Source: CAD feature listing. Evaluate the final solid. Frame: model axes, mm. Face numbers are marked on the shaded views. A direction names the side the tool comes from. Coordinates: 2 decimals unless noted, no trailing zeros. Order: outer loops, then holes, each group sorted by start corner. A loop starts at its lowest first (then second) coordinate and runs counter-clockwise, first axis right, second up.
Item 1: Section C-C on z = 28.25. Return the cut outline in (x, y), then the cut area to 3 significant figures.
Item 2: Contact query for flat-ended pins moving along their axis: P1, Ø0.8, axis at x = 15, y = 6.5, coming from the +Z side; P2, Ø1, axis at y = 9, z = 17.5, coming from the +X side; P3, Ø1, axis at x = 15.5, y = 9, coming from the -Z side. Output: stop coordinate, or through.
Item 3: Ray query, line 1 (X direction, y = 8, z = 8); line 2 (Z direction, x = 13.25, y = 6.8); line 3 (Z direction, x = 17.75, y = 8.85). Return the intervals inside material, ascending.
Item 4: Reachability of the marked faces 4, 5, 6 and 7 from +Z, -Z, +X, -X, +Y, -Y: full face, straight path, thin tool, end or side. Return the list, or none.
Item 5: Section B-B on x = 13.25. Return the cut outline in (y, z).
Item 6: Section A-A on y = 8.75. Return the cut outline in (x, z), then the cut area to 3 significant figures.
Item 7: Mould query, pull axis Y, two halves, no side actions, for the marked faces 1, 2 and 3. Classes: released by +Y, released by -Y, zero draft, split by the parting line, or undercut.
Item 8: Section D-D on y = 7.7. Return the cut outline in (x, z).
from build123d import *

# Parameters (mm, degrees)
CYLINDER_R     = 1.5
CYLINDER_DEPTH = 10
BOX004_W       = 1
BOX004_H       = 3
BOX004_DEPTH   = 3
BOX005_W       = 1
BOX005_H       = 3
BOX005_DEPTH   = 3
BOX006_W       = 6
BOX006_H       = 1
BOX006_DEPTH   = 3
BOX007_W       = 6
BOX007_H       = 1
BOX007_DEPTH   = 3
BOX003_W       = 6
BOX003_H       = 3.5
BOX003_DEPTH   = 20


with BuildPart() as cylinder:
    # Cylinder → Cylinder (new body)
    with BuildSketch(Plane(origin=(15, 8.75, 20), x_dir=(1, 0, 0), z_dir=(0, 0, 1))):
        Circle(CYLINDER_R)
    extrude(amount=CYLINDER_DEPTH)


with BuildPart() as box004:
    # Box004 → Box004 (new body)
    with BuildSketch(Plane(origin=(11, 7.25, 7), x_dir=(1, 0, 0), z_dir=(0, 0, 1))):
        with Locations((0.5, 1.5)):
            Rectangle(BOX004_W, BOX004_H)
    extrude(amount=BOX004_DEPTH)


with BuildPart() as box005:
    # Box005 → Box005 (new body)
    with BuildSketch(Plane(origin=(18, 7.25, 7), x_dir=(1, 0, 0), z_dir=(0, 0, 1))):
        with Locations((0.5, 1.5)):
            Rectangle(BOX005_W, BOX005_H)
    extrude(amount=BOX005_DEPTH)


with BuildPart() as box006:
    # Box006 → Box006 (new body)
    with BuildSketch(Plane(origin=(12, 6, 7), x_dir=(1, 0, 0), z_dir=(0, 0, 1))):
        with Locations((3, 0.5)):
            Rectangle(BOX006_W, BOX006_H)
    extrude(amount=BOX006_DEPTH)


with BuildPart() as box007:
    # Box007 → Box007 (new body)
    with BuildSketch(Plane(origin=(12, 10.5, 7), x_dir=(1, 0, 0), z_dir=(0, 0, 1))):
        with Locations((3, 0.5)):
            Rectangle(BOX007_W, BOX007_H)
    extrude(amount=BOX007_DEPTH)


with BuildPart() as bt_ex1:
    # Box003 → Box003 (new body)
    with BuildSketch(Plane(origin=(12, 7, 9), x_dir=(1, 0, 0), z_dir=(0, 0, 1))):
        with Locations((3, 1.75)):
            Rectangle(BOX003_W, BOX003_H)
    extrude(amount=BOX003_DEPTH)

    # Fusion: union Box004, Box005, Box006, Box007
    add(box004.part)
    add(box005.part)
    add(box006.part)
    add(box007.part)

    # Fusion005: union Cylinder
    add(cylinder.part)


solid = bt_ex1.part
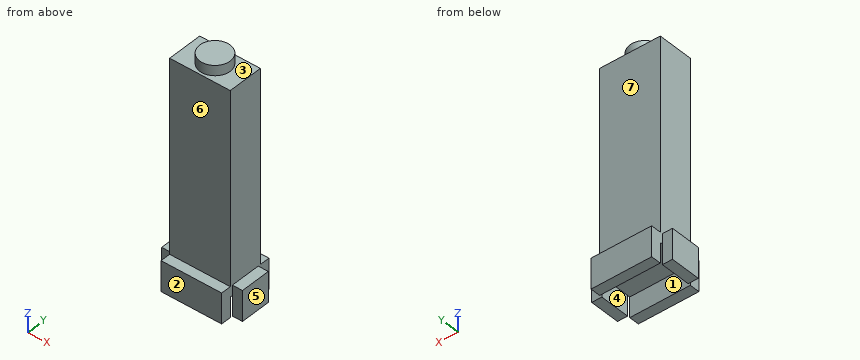
Answer list:
1. outline: (12, 7) - (18, 7) - (18, 10.5) - (12, 10.5) - close
1. area: 21.0 mm2
2. P1: stops at z = 10
2. P2: stops at x = 18
2. P3: stops at z = 9
3. line 1: x = 11 to 12, 18 to 19
3. line 2: z = 7 to 10
3. line 3: z = 9 to 29
4. face 4: -Z
4. face 5: +Z, -Z, +X, +Y, -Y
4. face 6: +Z, +X, -X, -Y
4. face 7: +Z, +X, -X, +Y
5. outline: (6, 7) - (7, 7) - (7, 9) - (10.5, 9) - (10.5, 7) - (11.5, 7) - (11.5, 10) - (10.5, 10) - (10.5, 29) - (7, 29) - (7, 10) - (6, 10) - close
6. outline: (11, 7) - (12, 7) - (12, 9) - (18, 9) - (18, 7) - (19, 7) - (19, 10) - (18, 10) - (18, 29) - (16.5, 29) - (16.5, 30) - (13.5, 30) - (13.5, 29) - (12, 29) - (12, 10) - (11, 10) - close
6. area: 129 mm2
7. face 1: undercut
7. face 2: released by -Y
7. face 3: zero draft
8. outline: (11, 7) - (12, 7) - (12, 9) - (18, 9) - (18, 7) - (19, 7) - (19, 10) - (18, 10) - (18, 29) - (16.07, 29) - (16.07, 30) - (13.93, 30) - (13.93, 29) - (12, 29) - (12, 10) - (11, 10) - close
